Here's how the part is built. I have some questions about the finished solid (model axes, mm). Round coordinates to 2 decimals unless told otherwise and drop trailing zeros. Write each loop counter-clockwise with the first axis right and the second up, starting at its lowest first coordinate (ties: lowest second). Pieces come first, ordered by that corner, then holes. Notation, with made-up numbers: (37.5, -14) - (68.5, -14) arc R11 ccw to (68.5, -6) - close; hole circle Ø1 at (-28, 64.25). An arc over 180 degrees is marked (long way). Return JSON: item names as keys, results as strings. Group by question number.
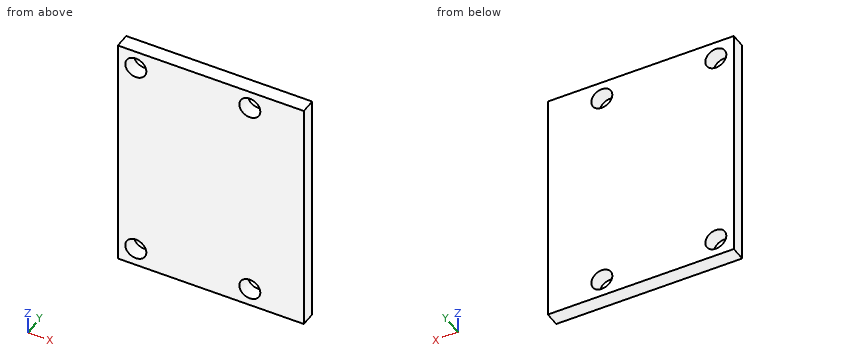
```python
from build123d import *

# Parameters (mm, degrees)
BOSS_EXTRUDE1_DEPTH = 40
CUT_EXTRUDE2_REACH  = 4.5
SKETCH3_R           = 1.75


with BuildPart() as part:
    # Sketch1 → Boss-Extrude1 (new body)
    with BuildSketch(Plane.XY):
        Polygon((0, 0), (-31, 0), (-31, 2.5), (-6, 2.5), (0, 2.5), align=None)
    extrude(amount=BOSS_EXTRUDE1_DEPTH)

    # Sketch3 → Cut-Extrude2 (cut, up to next)
    with BuildSketch(Plane(origin=(0, 2.5, 0), x_dir=(1, 0, 0), z_dir=(0, 1, 0)), mode=Mode.PRIVATE) as cut_extrude2_sk1:
        with Locations((-9, -3)):
            Circle(SKETCH3_R)
    cut_extrude2_tool1 = extrude(cut_extrude2_sk1.sketch, amount=-CUT_EXTRUDE2_REACH, mode=Mode.PRIVATE) & part.part
    add(cut_extrude2_tool1.solids().sort_by_distance((-9, 2.5, 3))[0], mode=Mode.SUBTRACT)
    # Sketch3 → Cut-Extrude2 (cut, up to next)
    with BuildSketch(Plane(origin=(0, 2.5, 0), x_dir=(1, 0, 0), z_dir=(0, 1, 0)), mode=Mode.PRIVATE) as cut_extrude2_sk2:
        with Locations((-28, -3)):
            Circle(SKETCH3_R)
    cut_extrude2_tool2 = extrude(cut_extrude2_sk2.sketch, amount=-CUT_EXTRUDE2_REACH, mode=Mode.PRIVATE) & part.part
    add(cut_extrude2_tool2.solids().sort_by_distance((-28, 2.5, 3))[0], mode=Mode.SUBTRACT)
    # Sketch3 → Cut-Extrude2 (cut, up to next)
    with BuildSketch(Plane(origin=(0, 2.5, 0), x_dir=(1, 0, 0), z_dir=(0, 1, 0)), mode=Mode.PRIVATE) as cut_extrude2_sk3:
        with Locations((-28, -37)):
            Circle(SKETCH3_R)
    cut_extrude2_tool3 = extrude(cut_extrude2_sk3.sketch, amount=-CUT_EXTRUDE2_REACH, mode=Mode.PRIVATE) & part.part
    add(cut_extrude2_tool3.solids().sort_by_distance((-28, 2.5, 37))[0], mode=Mode.SUBTRACT)
    # Sketch3 → Cut-Extrude2 (cut, up to next)
    with BuildSketch(Plane(origin=(0, 2.5, 0), x_dir=(1, 0, 0), z_dir=(0, 1, 0)), mode=Mode.PRIVATE) as cut_extrude2_sk4:
        with Locations((-9, -37)):
            Circle(SKETCH3_R)
    cut_extrude2_tool4 = extrude(cut_extrude2_sk4.sketch, amount=-CUT_EXTRUDE2_REACH, mode=Mode.PRIVATE) & part.part
    add(cut_extrude2_tool4.solids().sort_by_distance((-9, 2.5, 37))[0], mode=Mode.SUBTRACT)


solid = part.part
```
1) I need wall thicknesses on line 1 along Z through (x, y) = (-28, 1.9); line 2 along X through (y, z) = (0.95, 36.5); line 3 along Z through (x, y) = (-10, 1.75). Which ranges of each line are inside material? Lowest first, please.
2) Imagine slicing it at C-C (z = 3). Please give me the cut outline in (x, y).
3) Imagine slicing it at A-A (x = -9). Please give me the cut outline in (y, z), plus the area to 3 significant figures.
4) Imagine slicing it at B-B (y = 1.45). Please give me the cut outline in (x, z), plus the area to 3 significant figures.
5) Will this pin go through, and if not, where does the flat tip stop? pin 1 Ø6 at (x, z) = (-28, 21) entering from -Y.
Results found:
{
 "1": {"line 1": "z = 0 to 1.25, 4.75 to 35.25, 38.75 to 40", "line 2": "x = -31 to -29.68, -26.32 to -10.68, -7.32 to 0", "line 3": "z = 0 to 1.56, 4.44 to 35.56, 38.44 to 40"},
 "2": {"outline": "(-31, 0) - (-29.75, 0) - (-29.75, 2.5) - (-31, 2.5) - close; (-26.25, 0) - (-10.75, 0) - (-10.75, 2.5) - (-26.25, 2.5) - close; (-7.25, 0) - (0, 0) - (0, 2.5) - (-7.25, 2.5) - close"},
 "3": {"outline": "(0, 0) - (2.5, 0) - (2.5, 1.25) - (0, 1.25) - close; (0, 4.75) - (2.5, 4.75) - (2.5, 35.25) - (0, 35.25) - close; (0, 38.75) - (2.5, 38.75) - (2.5, 40) - (0, 40) - close", "area": "82.5 mm²"},
 "4": {"outline": "(-31, 0) - (0, 0) - (0, 40) - (-31, 40) - close; hole circle Ø3.5 at (-28, 3); hole circle Ø3.5 at (-28, 37); hole circle Ø3.5 at (-9, 3); hole circle Ø3.5 at (-9, 37)", "area": "1,200 mm²"},
 "5": {"pin 1": "stops at y = 0"}
}
